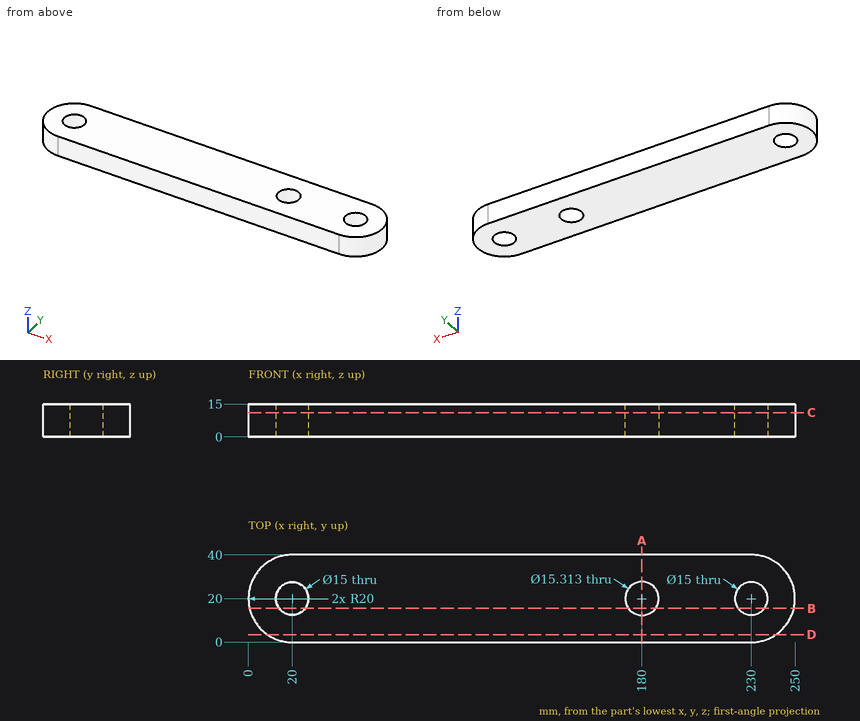
Check sheet for the drawn part. Datum: minimum x, y, z corner. Units: mm. Give positions to 0.01 mm unless a question says otherwise; leave off trailing zeros. Write each loop counter-clockwise with the first axis right and the second up, starting at its lowest first coordinate (ties: lowest second). Pieces come first, ordered by that corner, then holes. Notation, with made-up numbers: (2.25, -31.75) - (36.25, -31.75) arc R13 cw to (36.25, -15.75) - close; hole circle Ø5 at (28, 87). An arc over 180 degrees is marked (long way). Put each result on its own line as item: value.
1. Go/stop test with flat-tipped pins: pin 1 (13.5 mm diameter, centred on x = 20, y = 20, fed in from +Z); pin 2 (6 mm diameter, centred on y = 11.5, z = 12.5, fed in from +X); pin 3 (5 mm diameter, centred on y = 21, z = 11, fed in from +X); pin 4 (3 mm diameter, centred on y = 34.5, z = 11.5, fed in from +X). Record where each tip stops, or that it passes through.
Ans:
pin 1: passes through
pin 2: stops at x = 249.23
pin 3: stops at x = 250
pin 4: stops at x = 245.2
2. Sectioned sample at A-A, the plane x = 180. Enter the section's corners in (y, z).
Ans:
outline: (0, 0) - (12.34, 0) - (12.34, 15) - (0, 15) - close; (27.66, 0) - (40, 0) - (40, 15) - (27.66, 15) - close
3. Thickness scan on line 1 (Y direction, x = 230, z = 4); line 2 (Y direction, x = 180, z = 7.5); line 3 (X direction, y = 19, z = 9.5) (1 decimal). Record the ranges inside material, lowest first.
Ans:
line 1: y = 0 to 12.5, 27.5 to 40
line 2: y = 0 to 12.34, 27.66 to 40
line 3: x = 0 to 12.6, 27.4 to 172.4, 187.6 to 222.6, 237.4 to 250
4. Sectioned sample at B-B, the plane y = 15.5. Enter the section's corners in (x, z) (1 decimal), plus the area to 3 significant figures.
Ans:
outline: (0.5, 0) - (14, 0) - (14, 15) - (0.5, 15) - close; (26, 0) - (173.8, 0) - (173.8, 15) - (26, 15) - close; (186.2, 0) - (224, 0) - (224, 15) - (186.2, 15) - close; (236, 0) - (249.5, 0) - (249.5, 15) - (236, 15) - close
area: 3,190 mm²
5. Sectioned sample at D-D, the plane y = 3.5. Enter the section's corners in (x, z).
Ans:
outline: (8.7, 0) - (241.3, 0) - (241.3, 15) - (8.7, 15) - close
6. Sectioned sample at C-C, the plane z = 11. Enter the section's corners in (x, y), plus the area to 3 significant figures.
Ans:
outline: (20, 0) - (230, 0) arc R20 ccw to (230, 40) - (20, 40) arc R20 ccw to start; hole circle Ø15 at (20, 20); hole circle Ø15.31 at (180, 20); hole circle Ø15 at (230, 20)
area: 9,120 mm²
